Autodesk Inventor part; units mm, degrees
ref_plane "YZ Plane" through (0, 0, 0) normal (1, 0, 0) x (0, 1, 0)
ref_plane "XZ Plane" through (0, 0, 0) normal (0, 1, 0) x (-1, 0, 0)
ref_plane "XY Plane" through (0, 0, 0) normal (0, 0, 1) x (1, 0, 0)
sketch "Sketch1" plane through (0, 0, 0) normal (0, 1, 0) x (-1, 0, 0)
  circle A0 centre (0, 0) radius 77.47
  circle A1 centre (0, 0) radius 13.97
  dimension "d0" = 154.94
  dimension "d1" = 27.94
extrude "Extrusion1" add sketch "Sketch1" along normal blind 19.05
fillet "Fillet1" radius 9.525 2 edges at (77.47, 19.05, 0) (77.47, 0, 0)
chamfer "Chamfer1" distance 0.635 angle 45 2 edges at (13.97, 19.05, 0) (13.97, 0, 0)
properties part number "5lb_weight" material "Iron, Cast"
Could you check a few things on this model? Use its own coordinates, in mm. Round coordinates to 2 decimals unless told otherwise and drop trailing zeros. Loops run counter-clockwise (first coordinate to the right, second up) from the corner with the lowest first, then second, coordinate; pieces in that order, holes last. Notation, with made-up numbers: (51.5, 60) - (74.5, 60) arc R12 ccw to (74.5, 69) - close; hole circle Ø4 at (48, -33). An arc over 180 degrees is marked (long way). Answer in a Markdown table with one row per item. Add a question column.
(1) If we section it at C-C (y = 7.5): Please give me the cut outline in (x, z).
(2) I need wall thicknesses on line 1 along Z through (x, y) = (0, 9); line 2 along Z through (x, y) = (0, 9.75); line 3 along X through (y, z) = (7.5, 6.5). Which ranges of each line are inside material? Lowest first, please.
(3) If we mould it in two halves opening along Z, with no side actions, what happens to faces 1 (the face through (1, 0, 16)), 2 (the face through (1.82, 9.4, -13.85))? For each: pulls with the +Z half, pulls with the -Z half, needs draft (parallel to the pull), parting line crosses it, or undercut.
(4) If we section it at D-D (y = 15.5): Please give me the cut outline in (x, z).
(5) I'm going to push flat-ended pins straight in: pin 1 (1 mm diameter, centred on y = 2, z = 50.5, fed in from -X); pin 2 (4 mm diameter, centred on x = 50.5, z = -54, fed in from +Y); pin 3 (4 mm diameter, centred on x = -59.5, y = 16.5, fed in from +Z). Where does each tip first touch, or does it pass through?
Model answer:
| question | item | result |
|---|---|---|
| 1 | outline | circle Ø154.5 at (0, 0); hole circle Ø27.94 at (0, 0) |
| 2 | line 1 | z = -77.46 to -13.97, 13.97 to 77.46 |
| 2 | line 2 | z = -77.47 to -13.97, 13.97 to 77.47 |
| 2 | line 3 | x = -76.98 to -12.37, 12.37 to 76.98 |
| 3 | face 1 | needs draft |
| 3 | face 2 | undercut |
| 4 | outline | circle Ø150.73 at (0, 0); hole circle Ø27.94 at (0, 0) |
| 5 | pin 1 | stops at x = -54.74 |
| 5 | pin 2 | stops at y = 18.17 |
| 5 | pin 3 | stops at z = 48.51 |
